from build123d import *

# Parameters (mm, degrees)
BOSS_EXTRUDE1_DEPTH = 38.1
SKETCH2_R           = 7.14375
CUT_EXTRUDE1_DEPTH  = 89.488543914
SKETCH3_R           = 7.14375
CUT_EXTRUDE2_DEPTH  = 73.398431641


with BuildPart() as part:
    # Sketch1 → Boss-Extrude1 (new, symmetric)
    with BuildSketch(Plane.XY):
        with BuildLine():
            Line((-23.0251, -12.7), (-23.0251, -54.102))
            Line((-23.0251, -54.102), (-29.3751, -54.102))
            Line((-29.3751, -54.102), (-29.3751, -12.7))
            ThreePointArc((-29.3751, -12.7), (-25.655356121, -3.719743879), (-16.6751, 0))
            Line((-16.6751, 0), (16.6751, 0))
            ThreePointArc((16.6751, 0), (25.655356121, -3.719743879), (29.3751, -12.7))
            Line((29.3751, -12.7), (29.3751, -54.102))
            Line((29.3751, -54.102), (23.0251, -54.102))
            Line((23.0251, -54.102), (23.0251, -12.7))
            ThreePointArc((23.0251, -12.7), (21.165228061, -8.209871939), (16.6751, -6.35))
            Line((16.6751, -6.35), (-16.6751, -6.35))
            ThreePointArc((-16.6751, -6.35), (-21.165228061, -8.209871939), (-23.0251, -12.7))
        make_face()
    extrude(amount=BOSS_EXTRUDE1_DEPTH, both=True)

    # Sketch2 → Cut-Extrude1 (cut, through all)
    with BuildSketch(Plane(origin=(29.3751, 0, 0), x_dir=(0, 0, -1), z_dir=(1, 0, 0))):
        with Locations(Location((0, -38.1, 0), (0, 0, 90))):
            Circle(SKETCH2_R)
    extrude(amount=-CUT_EXTRUDE1_DEPTH, mode=Mode.SUBTRACT)

    # Sketch3 → Cut-Extrude2 (cut, through all)
    with BuildSketch(Plane(origin=(0, 0, 0), x_dir=(1, 0, 0), z_dir=(0, 1, 0))):
        with Locations(Location((0, 22.86, 0), (0, 0, 270))):
            Circle(SKETCH3_R)
        with Locations(Location((0, -22.86, 0), (0, 0, 270))):
            Circle(SKETCH3_R)
    extrude(amount=-CUT_EXTRUDE2_DEPTH, mode=Mode.SUBTRACT)


solid = part.part
Can you work these out from the model? Positions are in its coordinate system, mm. A direction names the side the tool comes from. Coordinates: 2 decimals unless noted, no trailing zeros. Write each loop counter-clockwise with the first axis right and the second up, starting at its lowest first coordinate (ties: lowest second). Pieces come first, ordered by that corner, then holes. Notation, with made-up numbers: (-35.75, 26.25) -> (-9.75, 26.25) arc R21 cw to (-9.75, 38.25) -> close; hole circle Ø9 at (-26.75, 7.5). An arc over 180 degrees is marked (long way). Write each question's results on one line, items separated by ' | '. Start each with the question number.
Q1. I'm going to push flat-ended pins straight in: pin 1 (1.5 mm diameter, centred on y = -5.5, z = -15, fed in from -X); pin 2 (23 mm diameter, centred on x = 0, z = -22.86, fed in from -Y); pin 3 (11.5 mm diameter, centred on y = -38.1, z = 0, fed in from +X). Where does each tip first touch, or does it pass through?
Q2. Imagine slicing it at C-C (y = -38.1). Write out the boundary of the cut face in (x, z).
Q3. Imagine slicing it at A-A (z = -22.86). Write out the boundary of the cut face in (x, y), then the cut area to 3 significant figures.
Q4. On a 3-axis mill with a long thin cutter (end or side, diameter ignored), from which of +Z, -Z, +X, -X, +Y, -Y can I reach the whole of each face in a straight line? I mean faces 4 (the face through (0.314, -3.131, -29.997)), 5 (the face through (21.214, -8.26, 0.533)). Say none if no direction works.
Q5. If I drill on probe 1 along X at (y, z) = (-50, -7); probe 2 along Z at (x, y) = (-27.5, -38.1); probe 3 along X at (y, z) = (-5, 22.86), over which ranges is the centre line in solid material (lowest first)?
Q6. We'd pull the mould along Y, two halves only. Please class faces 1 (the face through (-25.754, -3.819, 0.533)), 2 (the face through (-26, -54.102, 1)), 3 (the face through (-26.156, -45.237, 0.314)): +Y half, -Y half, draft (parallel to the pull), parting line (faces both ways), or undercut.
Q7. Imagine slicing it at D-D (z = 0). Write out the boundary of the cut face in (x, y), then the cut area to 3 significant figures.
Q8. Imagine slicing it at B-B (x = 0). Write out the boundary of the cut face in (y, z).
Taken from the geometry:
1) pin 1: stops at x = -27.62 | pin 2: stops at y = -6.35 | pin 3: passes through
2) outline: (-29.38, -38.1) -> (-23.03, -38.1) -> (-23.03, -7.14) -> (-29.38, -7.14) -> close; (-29.38, 7.14) -> (-23.03, 7.14) -> (-23.03, 38.1) -> (-29.38, 38.1) -> close; (23.03, -38.1) -> (29.38, -38.1) -> (29.38, -7.14) -> (23.03, -7.14) -> close; (23.03, 7.14) -> (29.38, 7.14) -> (29.38, 38.1) -> (23.03, 38.1) -> close
3) outline: (-29.38, -54.1) -> (-23.03, -54.1) -> (-23.03, -12.7) arc R6.35 cw to (-16.68, -6.35) -> (-7.14, -6.35) -> (-7.14, 0) -> (-16.68, 0) arc R12.7 ccw to (-29.38, -12.7) -> close; (7.14, -6.35) -> (16.68, -6.35) arc R6.35 cw to (23.03, -12.7) -> (23.03, -54.1) -> (29.38, -54.1) -> (29.38, -12.7) arc R12.7 ccw to (16.68, 0) -> (7.14, 0) -> close | area: 837 mm^2
4) face 4: +Y, -Y | face 5: +Z, -Z, -Y
5) probe 1: x = -29.38 to -23.03, 23.03 to 29.38 | probe 2: z = -38.1 to -7.14, 7.14 to 38.1 | probe 3: x = -26.77 to -7.14, 7.14 to 26.77
6) face 1: +Y half | face 2: -Y half | face 3: undercut
7) outline: (-29.38, -54.1) -> (-23.03, -54.1) -> (-23.03, -45.24) -> (-29.38, -45.24) -> close; (-29.38, -30.96) -> (-23.03, -30.96) -> (-23.03, -12.7) arc R6.35 cw to (-16.68, -6.35) -> (16.68, -6.35) arc R6.35 cw to (23.03, -12.7) -> (23.03, -30.96) -> (29.38, -30.96) -> (29.38, -12.7) arc R12.7 ccw to (16.68, 0) -> (-16.68, 0) arc R12.7 ccw to (-29.38, -12.7) -> close; (23.03, -54.1) -> (29.38, -54.1) -> (29.38, -45.24) -> (23.03, -45.24) -> close | area: 746 mm^2
8) outline: (-6.35, -38.1) -> (0, -38.1) -> (0, -30) -> (-6.35, -30) -> close; (-6.35, -15.72) -> (0, -15.72) -> (0, 15.72) -> (-6.35, 15.72) -> close; (-6.35, 30) -> (0, 30) -> (0, 38.1) -> (-6.35, 38.1) -> close
